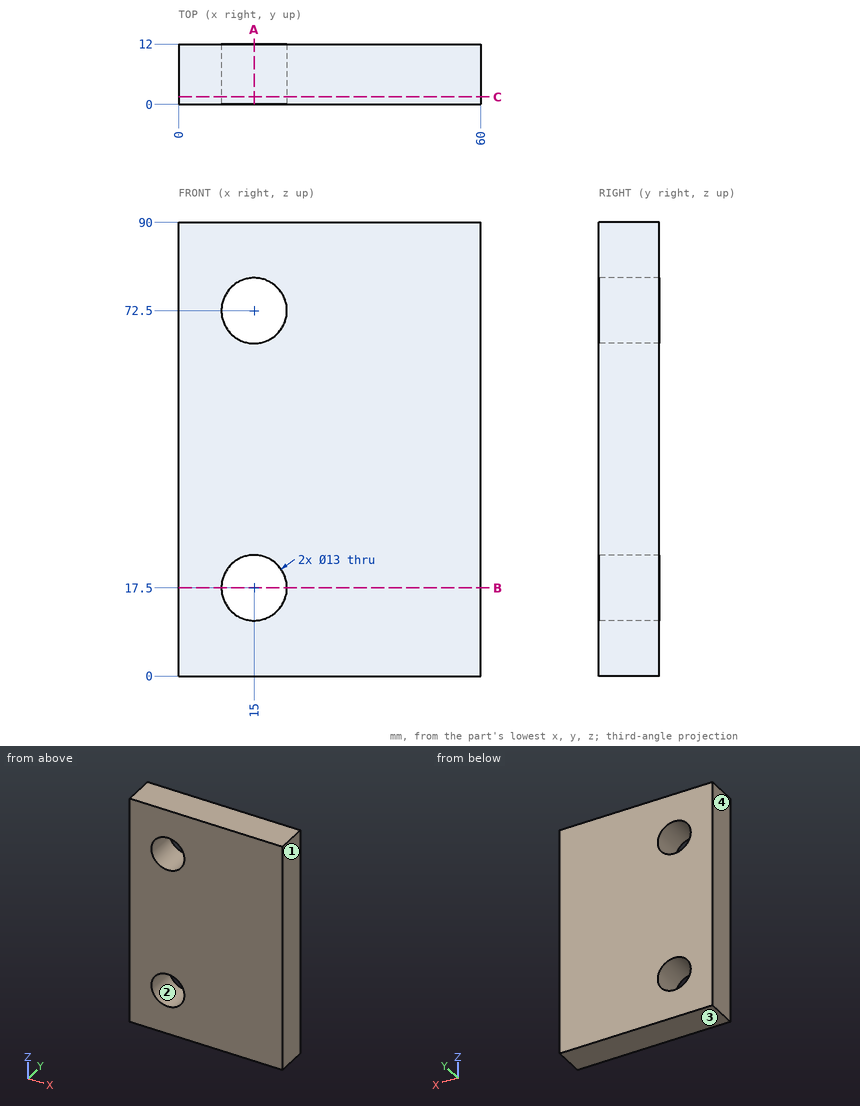
Source: three-view drawing plus pictorial views. Frame: mm from the lowest corner of the part. Give positions to 0.01 mm unless a question says otherwise; leave off trailing zeros. Order: outer loops, then holes, each group sorted by start corner. A loop starts at its lowest first (then second) coordinate and runs counter-clockwise, first axis right, second up. Notation, with made-up numbers: (-6, -26.75) -> (25, -26.75) arc R27 cw to (25, 5.25) -> close; hole circle Ø7 at (-16, 71.25). An arc over 180 degrees is marked (long way). Put each result on its own line as item: value.
Q1. Section C-C, the plane y = 1.5. Return loops of the section in (x, z), then the cut area to 3 significant figures.
Here are the results:
outline: (0, 0) -> (60, 0) -> (60, 90) -> (0, 90) -> close; hole circle Ø13 at (15, 17.5); hole circle Ø13 at (15, 72.5)
area: 5,130 mm^2
Q2. Section A-A, the plane x = 15. Return loops of the section in (y, z), then the cut area to 3 significant figures.
Here are the results:
outline: (0, 0) -> (12, 0) -> (12, 11) -> (0, 11) -> close; (0, 24) -> (12, 24) -> (12, 66) -> (0, 66) -> close; (0, 79) -> (12, 79) -> (12, 90) -> (0, 90) -> close
area: 768 mm^2
Q3. Draft query along X for the marked faces 1, 2, 3 and 4. Return one class per face: released by +X, released by -X, zero draft, split by the parting line, or undercut.
Here are the results:
face 1: released by +X
face 2: undercut
face 3: zero draft
face 4: released by -X
Q4. Section B-B, the plane z = 17.5. Return loops of the section in (x, y), then the cut area to 3 significant figures.
Here are the results:
outline: (0, 0) -> (8.5, 0) -> (8.5, 12) -> (0, 12) -> close; (21.5, 0) -> (60, 0) -> (60, 12) -> (21.5, 12) -> close
area: 564 mm^2
Q5. Material intervals for L1, parallel to Z at x = 15, y = 3.5; L2, parallel to X at y = 4.25, z = 72.5; L3, parallel to Z at x = 21, y = 3, sorted ascending.
Here are the results:
L1: z = 0 to 11, 24 to 66, 79 to 90
L2: x = 0 to 8.5, 21.5 to 60
L3: z = 0 to 15, 20 to 70, 75 to 90
